```python
from build123d import *

# Parameters (mm, degrees)
F0_R            = 38.1
F1_DEPTH        = 12.7
F4_DEPTH        = 3.175
F4_COPIES_COUNT = 20


# Not quite as in the source:
# - a pattern or mirror of a feature is missing from the dataset's text; its kind, count and spacing are read off the source's solid


with BuildPart() as f1:
    # F0 (on Front) → F1 (new body, symmetric)
    with BuildSketch(Plane.XZ):
        Circle(F0_R)
    extrude(amount=F1_DEPTH, both=True)

    # F3 (on offset) → F4 (cut)
    with BuildSketch(Plane.XY.offset(38.1)):
        Polygon((-6.8059094878, -12.7), (0, -12.7), (6.8059094878, 12.7), (0, 12.7), align=None)
    f4 = extrude(amount=-F4_DEPTH, mode=Mode.SUBTRACT)

    # F4_copies: F4 ×20 about axis
    f4_copies_axis = Axis((0, 0, 0), (0, 1, 0))
    for i in range(1, F4_COPIES_COUNT):
        add(f4.rotate(f4_copies_axis, i * 360 / F4_COPIES_COUNT), mode=Mode.SUBTRACT)


solid = f1.part
```
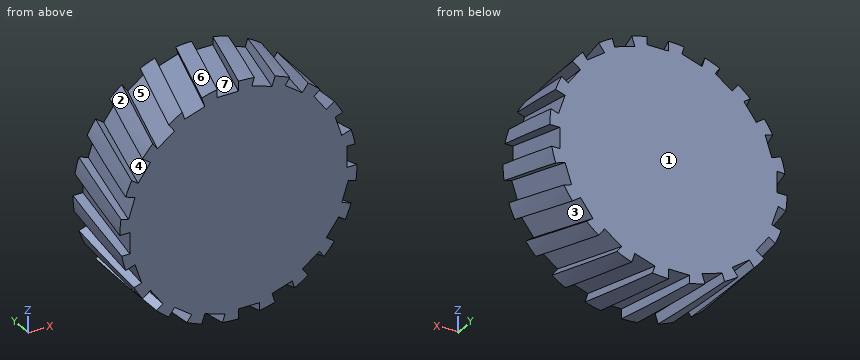
For this review, take the finished solid that the model builds, in its own axes (mm). Face numbers are marked on the shaded views. A direction names the side the tool comes from. Coordinates: 2 decimals unless noted, no trailing zeros. Loops run counter-clockwise (first coordinate to the right, second up) from the corner with the lowest first, then second, coordinate; pieces in that order, holes last.
1. Add section C-C, the plane z = 9.5. Give the boundary of the cut face in (x, y), then the cut area to 3 significant figures.
2. For line 1 (X direction, y = 8, z = 25.5); line 2 (Z direction, x = 5, y = -5.5); line 3 (X direction, y = 9.5, z = -20), list the stretches that pass through material, from the lowest coordinate up.
3. Insertion check: P1, Ø4, axis at y = -3.5, z = -1.5, coming from the +X side; P2, Ø15, axis at x = 3, y = 0, coming from the -Z side; P3, Ø4, axis at y = -8.5, z = 11, coming from the -X side. Each pin has a flat end and moves straight along its axis. Give the tip position at first contact, or say it passes through.
4. Mouldability with a two-part tool opening along X and no side actions: class the marked faces 1, 2, 3 and 4 as +X half, -X half, draft (parallel to the pull), parting line (faces both ways), or undercut.
5. Add section B-B, the plane x = 8. Give the boundary of the cut face in (y, z), then the cut area to 3 significant figures.
6. Add section A-A, the plane z = 21.5. Give the boundary of the cut face in (x, y), then the cut area to 3 significant figures.
7. For the marked faces 5, 6 and 7, list the 3-axis set-ups (+Z, -Z, +X, -X, +Y, -Y) from which the entire face can be reached by the end or side of a thin tool; tool diameter is ignored.
Result:
1. outline: (-36.9, 3.87) - (-33.64, 7.63) - (-33.64, -12.7) - (36.9, -12.7) - (36.9, -3.87) - (33.64, -7.63) - (33.64, 12.7) - (-36.9, 12.7) - close
1. area: 1,750 mm2
2. line 1: x = -25.66 to 24.32, 25.38 to 28.31
2. line 2: z = -37.77 to 37.77
2. line 3: x = -28.64 to 28.64, 28.99 to 32.43
3. P1: stops at x = 38.05
3. P2: stops at z = -38.07
3. P3: stops at x = -35.99
4. face 1: draft
4. face 2: -X half
4. face 3: undercut
4. face 4: undercut
5. outline: (-12.7, -37.25) - (1.86, -37.25) - (-1.74, -34.12) - (12.7, -34.12) - (12.7, 37.25) - (-1.86, 37.25) - (1.74, 34.12) - (-12.7, 34.12) - close
5. area: 1,810 mm2
6. outline: (-31.45, 8.62) - (-29.59, 12.7) - (-31.45, 12.7) - close; (-29.59, -12.7) - (27.55, -12.7) - (27.55, 8.22) - (29.59, 12.7) - (-27.55, 12.7) - (-27.55, -8.22) - close; (29.59, -12.7) - (31.45, -12.7) - (31.45, -8.62) - close
6. area: 1,420 mm2
7. face 5: none
7. face 6: +Z, -X, +Y, -Y
7. face 7: +Z
